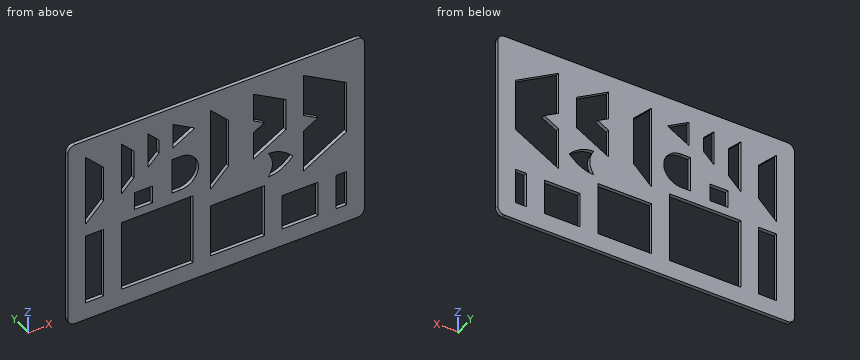
from build123d import *

# Parameters (mm, degrees)
SKETCH1_W           = 83
SKETCH1_H           = 53.635971978
SKETCH1_W_2         = 20
SKETCH1_H_2         = 20
SKETCH1_W_3         = 15
SKETCH1_H_3         = 15
SKETCH1_W_4         = 10
SKETCH1_H_4         = 10
SKETCH1_W_5         = 5
SKETCH1_W_6         = 3
SKETCH1_H_5         = 5
BOSS_EXTRUDE1_DEPTH = 1
FILLET1_R           = 2


with BuildPart() as part:
    # Sketch1 → Boss-Extrude1 (new body)
    with BuildSketch(Plane(origin=(0, 0, 0), x_dir=(1, 0, 0), z_dir=(0, 1, 0))):
        with Locations((-25.700677223, 6.877666185)):
            Rectangle(SKETCH1_W, SKETCH1_H)
        Polygon((-62.200677223, 5.059680196), (-62.200677223, -14.940319804), (-57.200677223, -9.940319804), (-57.200677223, 0.059680196), align=None, mode=Mode.SUBTRACT)
        with Locations((-42.200677223, 18.695652174)):
            Rectangle(SKETCH1_W_2, SKETCH1_H_2, mode=Mode.SUBTRACT)
        with Locations((-19.700677223, 21.195652174)):
            Rectangle(SKETCH1_W_3, SKETCH1_H_3, mode=Mode.SUBTRACT)
        with Locations((-2.200677223, 23.695652174)):
            Rectangle(SKETCH1_W_4, SKETCH1_H_4, mode=Mode.SUBTRACT)
        with Locations((-59.700677223, 18.695652174)):
            Rectangle(SKETCH1_W_5, SKETCH1_H_2, mode=Mode.SUBTRACT)
        with Locations((9.299322777, 23.695652174)):
            Rectangle(SKETCH1_W_6, SKETCH1_H_4, mode=Mode.SUBTRACT)
        Polygon((-52.200677223, -14.940319804), (-52.200677223, 0.059680196), (-48.700677223, -3.440319804), (-48.700677223, -11.440319804), align=None, mode=Mode.SUBTRACT)
        Polygon((-44.700677223, -4.940319804), (-44.700677223, -14.940319804), (-41.700677223, -11.940319804), (-41.700677223, -7.940319804), align=None, mode=Mode.SUBTRACT)
        Polygon((-1.200677223, 13.67848235), (-1.200677223, 1.67848235), (2.799322777, -0.630918727), (-1.200677223, -2.940319804), (-1.200677223, -14.940319804), (10.799322777, -8.012116573), (10.799322777, 6.750279119), align=None, mode=Mode.SUBTRACT)
        Polygon((-15.200677223, 4.523781811), (-15.200677223, -3.476218189), (-12.200677223, -5.208268996), (-15.200677223, -6.940319804), (-15.200677223, -14.940319804), (-6.200677223, -9.744167381), (-6.200677223, -0.672370611), align=None, mode=Mode.SUBTRACT)
        Polygon((-27.200677223, 8.695652174), (-27.200677223, -14.940319804), (-22.200677223, -9.940319804), (-22.200677223, 3.695652174), align=None, mode=Mode.SUBTRACT)
        Polygon((-37.700677223, -14.940319804), (-37.700677223, -7.940319804), (-31.638499397, -11.440319804), align=None, mode=Mode.SUBTRACT)
        with Locations((-46.067733945, 3.695652174)):
            Rectangle(SKETCH1_W_5, SKETCH1_H_5, mode=Mode.SUBTRACT)
        with BuildLine():
            Line((-35.634253982, 5.478469437), (-38.073838133, 5.478469437))
            Line((-38.073838133, 5.478469437), (-38.073838133, -4.521530563))
            Line((-38.073838133, -4.521530563), (-35.634253982, -4.521530563))
            ThreePointArc((-35.634253982, -4.521530563), (-30.634253982, 0.478469437), (-35.634253982, 5.478469437))
        make_face(mode=Mode.SUBTRACT)
        with BuildLine():
            add(Edge.make_bspline(
                [(-11.041888769, 11.517886634), (-8.809163486, 8.017886634), (-11.041888769, 4.517886634)],
                knots=[0, 0, 0, 1, 1, 1], degree=2))
            add(Edge.make_bspline(
                [(-11.041888769, 4.517886634), (-7.404142371, 4.517886634), (-4.201433986, 8.017886634)],
                knots=[0, 0, 0, 1, 1, 1], degree=2))
            add(Edge.make_bspline(
                [(-11.041888769, 11.517886634), (-7.453218548, 11.517886634), (-4.201433986, 8.017886634)],
                knots=[0, 0, 0, 1, 1, 1], degree=2))
        make_face(mode=Mode.SUBTRACT)
    extrude(amount=BOSS_EXTRUDE1_DEPTH)

    # Fillet1
    fillet1_edges = [part.edges().sort_by_distance(p)[0] for p in [
        (-67.200677223, 0.5, -33.695652174),
        (15.799322777, 0.5, -33.695652174),
        (15.799322777, 0.5, 19.940319804),
        (-67.200677223, 0.5, 19.940319804),
    ]]
    fillet(fillet1_edges, radius=FILLET1_R)


solid = part.part
The model under review builds one solid part; all positions refer to its coordinate system, in mm. Give positions to 0.01 mm unless a question says otherwise; leave off trailing zeros. Loops run counter-clockwise (first coordinate to the right, second up) from the corner with the lowest first, then second, coordinate; pieces in that order, holes last. Notation, with made-up numbers: (-36.5, -31) -> (-17.5, -31) arc R32 cw to (-17.5, -3) -> close; hole circle Ø2 at (43, 83). An arc over 180 degrees is marked (long way). Answer as a JSON object with one key per item and string values. Group by question number.
Q1. Take a section at B-B (x = -19.5). Write out the cut boundary in (y, z), plus the area to 3 significant figures.
Q2. Take a section at A-A (z = -25.5). Write out the cut boundary in (x, y).
Q3. Wall thickness on line 1 along X through (y, z) = (0.6, -17); line 2 along Z through (x, y) = (-47, 0.7); line 3 along Z through (x, y) = (-21.5, 0.8): over which ranges is each line inside the solid? List them lowest first.
Q4. Take a section at D-D (y = 0.6). State how many separate pieces and enclosed holes the cut face has, plus the area to 3 significant figures.
Q5. Take a section at C-C (x = -34). Write out the cut boundary in (y, z), plus the area to 3 significant figures.
Answer below:
{
 "1": {"outline": "(0, -33.7) -> (1, -33.7) -> (1, -28.7) -> (0, -28.7) -> close; (0, -13.7) -> (1, -13.7) -> (1, 19.94) -> (0, 19.94) -> close", "area": "38.6 mm2"},
 "2": {"outline": "(-67.2, 0) -> (-62.2, 0) -> (-62.2, 1) -> (-67.2, 1) -> close; (-57.2, 0) -> (-52.2, 0) -> (-52.2, 1) -> (-57.2, 1) -> close; (-32.2, 0) -> (-27.2, 0) -> (-27.2, 1) -> (-32.2, 1) -> close; (-12.2, 0) -> (-7.2, 0) -> (-7.2, 1) -> (-12.2, 1) -> close; (2.8, 0) -> (7.8, 0) -> (7.8, 1) -> (2.8, 1) -> close; (10.8, 0) -> (15.8, 0) -> (15.8, 1) -> (10.8, 1) -> close"},
 "3": {"line 1": "x = -67.2 to -62.2, -57.2 to -52.2, -32.2 to -27.2, -12.2 to 15.8", "line 2": "z = -33.7 to -28.7, -8.7 to -6.2, -1.2 to 19.94", "line 3": "z = -33.7 to -28.7, -13.7 to 19.94"},
 "4": {"separate pieces": "1", "enclosed holes": "15", "area": "2,850 mm2"},
 "5": {"outline": "(0, -33.7) -> (1, -33.7) -> (1, -28.7) -> (0, -28.7) -> close; (0, -8.7) -> (1, -8.7) -> (1, -5.2) -> (0, -5.2) -> close; (0, 4.25) -> (1, 4.25) -> (1, 10.08) -> (0, 10.08) -> close; (0, 12.8) -> (1, 12.8) -> (1, 19.94) -> (0, 19.94) -> close", "area": "21.5 mm2"}
}
